Input: part model. Units: mm. Frame: model coordinates. A direction names the side the tool comes from. Round coordinates to 2 decimals unless told otherwise and drop trailing zeros. Write each loop counter-clockwise with the first axis right and the second up, starting at its lowest first coordinate (ties: lowest second). Pieces come first, ordered by that corner, then holes. Notation, with made-up numbers: M 72,49.5 L 128,49.5 A24 cw 128,77.5 Z; hole C 71.5,63.5 d11. An arc over 180 degrees is marked long. Write each question's results on one line, items separated by ' | '. Start each with the question number.
```python
from build123d import *

# Parameters (mm, degrees)
SKETCH1_R                = 8.4375
SKETCH1_R_2              = 1.5
BOSS_EXTRUDE1_DEPTH      = 6.35
FILLET1_R                = 8
F_7_16_CLEARANCE_HOLE4_D = 11.50874
BOSS_EXTRUDE2_DEPTH      = 12.7
FILLET2_R                = 5


with BuildPart() as part:
    # Sketch1 → Boss-Extrude1 (new body, symmetric)
    with BuildSketch(Plane.XY):
        with BuildLine():
            Line((-28, 72.922835534), (-28, 90))
            ThreePointArc((-28, 90), (-25.656854249, 95.656854249), (-20, 98))
            Line((-20, 98), (-11.5, 98))
            ThreePointArc((-11.5, 98), (-9.378679656, 97.121320344), (-8.5, 95))
            Line((-8.5, 95), (-8.5, 81))
            Line((-8.5, 81), (8.5, 81))
            Line((8.5, 81), (8.5, 95))
            ThreePointArc((8.5, 95), (9.378679656, 97.121320344), (11.5, 98))
            Line((11.5, 98), (20, 98))
            ThreePointArc((20, 98), (25.656854249, 95.656854249), (28, 90))
            Line((28, 90), (28, 72.922835534))
            Line((28, 72.922835534), (15, 59.922835534))
            Line((15, 59.922835534), (15, -59.922835534))
            Line((15, -59.922835534), (28, -72.922835534))
            Line((28, -72.922835534), (28, -90))
            ThreePointArc((28, -90), (25.656854249, -95.656854249), (20, -98))
            Line((20, -98), (11.5, -98))
            ThreePointArc((11.5, -98), (9.378679656, -97.121320344), (8.5, -95))
            Line((8.5, -95), (8.5, -81))
            Line((8.5, -81), (-8.5, -81))
            Line((-8.5, -81), (-8.5, -95))
            ThreePointArc((-8.5, -95), (-9.378679656, -97.121320344), (-11.5, -98))
            Line((-11.5, -98), (-20, -98))
            ThreePointArc((-20, -98), (-25.656854249, -95.656854249), (-28, -90))
            Line((-28, -90), (-28, -72.922835534))
            Line((-28, -72.922835534), (-15, -59.922835534))
            Line((-15, -59.922835534), (-15, 59.922835534))
            Line((-15, 59.922835534), (-28, 72.922835534))
        make_face()
        Circle(SKETCH1_R, mode=Mode.SUBTRACT)
        with Locations((-20, 90)):
            Circle(SKETCH1_R_2, mode=Mode.SUBTRACT)
        with Locations((20, 90)):
            Circle(SKETCH1_R_2, mode=Mode.SUBTRACT)
        with Locations((20, -90)):
            Circle(SKETCH1_R_2, mode=Mode.SUBTRACT)
        with Locations((-20, -90)):
            Circle(SKETCH1_R_2, mode=Mode.SUBTRACT)
    extrude(amount=BOSS_EXTRUDE1_DEPTH, both=True)

    # Fillet1
    fillet1_edges = [part.edges().sort_by_distance(p)[0] for p in [
        (-28, 72.922835534, 0),
        (28, 72.922835534, 0),
        (15, 59.922835534, 0),
        (15, -59.922835534, 0),
        (28, -72.922835534, 0),
        (-28, -72.922835534, 0),
        (-15, -59.922835534, 0),
        (-15, 59.922835534, 0),
    ]]
    fillet(fillet1_edges, radius=FILLET1_R)

    # 7/16 Clearance Hole4 (through all)
    with Locations(Plane.XY.offset(6.35)):
        with Locations((0, 36.5125), (0, -36.5125)):
            Hole(F_7_16_CLEARANCE_HOLE4_D / 2)

    # Sketch6 → Boss-Extrude2 (add)
    with BuildSketch(Plane.XY.offset(6.35)):
        Polygon((-15, 30.340959615), (-23.8125, 15.4813), (-23.8125, -15.4813), (-15, -30.340959615), align=None)
        Polygon((23.8125, -15.4813), (15, -30.340959615), (15, 30.340959615), (23.8125, 15.4813), align=None)
    extrude(amount=-BOSS_EXTRUDE2_DEPTH)

    # Fillet2
    fillet2_edges = [part.edges().sort_by_distance(p)[0] for p in [
        (-23.8125, 15.4813, 0),
        (-23.8125, -15.4813, 0),
        (-15, -30.340959615, 0),
        (-15, 30.340959615, 0),
        (15, 30.340959615, 0),
        (15, -30.340959615, 0),
        (23.8125, -15.4813, 0),
        (23.8125, 15.4813, 0),
    ]]
    fillet(fillet2_edges, radius=FILLET2_R)


solid = part.part
```
1. Draft query along Y for faces 1 (the face through (-12, 1, 6.35)), 2 (the face through (21.558, 66.481, 0.089)), 3 (the face through (-25.719, 95.594, 0.089)). Return one class per face: +Y half, -Y half, draft (parallel to the pull), parting line (faces both ways), or undercut.
2. Contact query for flat-ended pins moving along their axis: P1, Ø2, axis at x = -17.5, y = -53, coming from the +Z side; P2, Ø4, axis at x = -2, z = -2, coming from the -Y side; P3, Ø6, axis at y = 40.5, z = 2.5, coming from the -X side; P4, Ø4, axis at x = 20, y = -90, coming from the -Z side. Output: stop coordinate, or through.
3. Access query for faces 4 (the face through (8.5, 88, 0)), 5 (the face through (15, -44, 0)), 6 (the face through (-19.354, 22.999, 0.089)). Directions: +Z, -Z, +X, -X, +Y, -Y. A direction counts if a zero-diameter tool reaches every point of the face in a straight line with its end or side. Return the directions, or none.
4. Cut plane B-B on z = -4.25. Give the number of separate pieces and of enclosed holes in the cut face, and give its area (3 significant figures).
5. Cut plane A-A on y = 0. Output: boundary loops of the cut face in (x, z).
6. Line query: L1, parallel to Y at x = 0, z = 3.25; L2, parallel to X at y = -90, z = -1.5; L3, parallel to Y at x = -17.5, z = -4. Output: solid intervals per line, ascending. Write a range as from..to.
Answers follow:
1) face 1: draft | face 2: undercut | face 3: +Y half
2) P1: passes through | P2: stops at y = -81 | P3: stops at x = -15 | P4: stops at z = -6.35
3) face 4: +Z, -Z, +Y | face 5: +Z, -Z, +X | face 6: +Z, -Z, -X
4) separate pieces: 1 | enclosed holes: 7 | area: 7,230 mm2
5) outline: M -23.81,-6.35 L -8.44,-6.35 L -8.44,6.35 L -23.81,6.35 Z; M 8.44,-6.35 L 23.81,-6.35 L 23.81,6.35 L 8.44,6.35 Z
6) L1: y = -81..-42.27, -30.76..-8.44, 8.44..30.76, 42.27..81 | L2: x = -28..-21.5, -18.5..-8.5, 8.5..18.5, 21.5..28 | L3: y = -98..-62.42, -26.13..26.13, 62.42..98
